Could you check a few things on this drawing? It's one solid part, dimensions in mm from its lowest x, y, z. Round coordinates to 2 decimals unless told otherwise and drop trailing zeros. Loops run counter-clockwise (first coordinate to the right, second up) from the corner with the lowest first, then second, coordinate; pieces in that order, holes last. Notation, with made-up numbers: (-32, 88.25) -> (-16, 88.25) arc R33 cw to (-16, 122.25) -> close; hole circle Ø10 at (30, 29.25). An arc over 180 degrees is marked (long way). Use one line per item in the form item = value. Start each with the question number.
Item 1: If I drill on L1, parallel to Y at x = 168, z = 8; L2, parallel to Y at x = 127.5, z = 19.25, over which ranges is the centre line in solid material (lowest first)? Write a range as [from, to].
Item 2: If we section it at C-C (x = 223): Write out the boundary of the cut face in (y, z), then the cut area to 3 significant figures.
Item 3: If we section it at A-A (y = 20.25): Write out the boundary of the cut face in (x, z).
Item 4: I'm going to push flat-ended pins straight in: pin 1 Ø0.6 at (x, z) = (140, 23.5) entering from +Y; pin 2 Ø6 at (y, z) = (19.5, 14.5) entering from +X. Where does each tip first touch, or does it pass through?
Item 5: If we section it at D-D (y = 4.75): Write out the boundary of the cut face in (x, z).
Item 6: If we section it at B-B (z = 11): Write out the boundary of the cut face in (x, y), then the cut area to 3 significant figures.
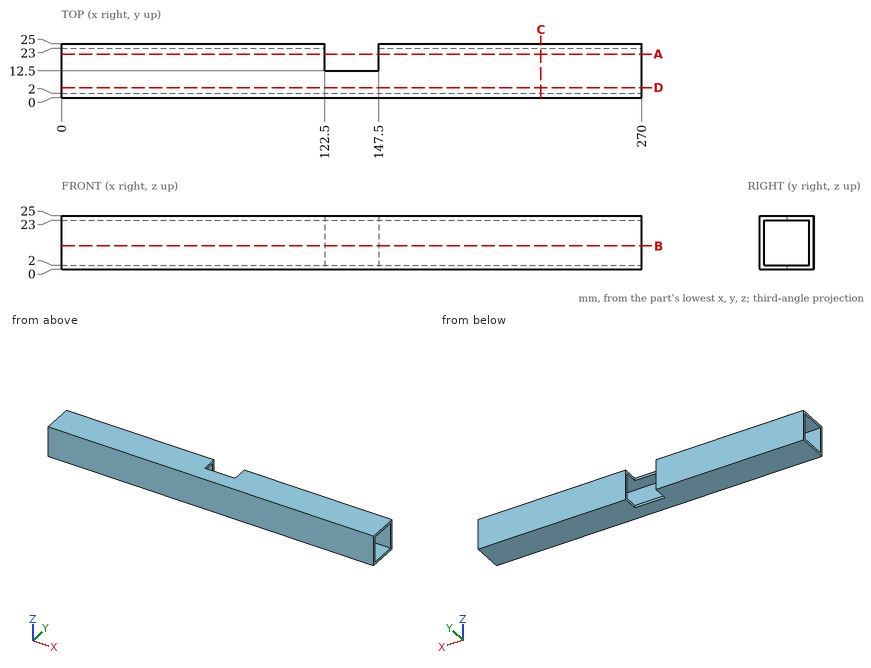
Values found:
q1.L1 = [0, 2], [23, 25]
q1.L2 = [0, 2]
q2.outline = (0, 0) -> (25, 0) -> (25, 25) -> (0, 25) -> close; hole (2, 2) -> (23, 2) -> (23, 23) -> (2, 23) -> close
q2.area = 184 mm2
q3.outline = (0, 0) -> (122.5, 0) -> (122.5, 2) -> (0, 2) -> close; (0, 23) -> (122.5, 23) -> (122.5, 25) -> (0, 25) -> close; (147.5, 0) -> (270, 0) -> (270, 2) -> (147.5, 2) -> close; (147.5, 23) -> (270, 23) -> (270, 25) -> (147.5, 25) -> close
q4.pin_1 = 12.5
q4.pin_2 = through
q5.outline = (0, 0) -> (270, 0) -> (270, 2) -> (0, 2) -> close; (0, 23) -> (270, 23) -> (270, 25) -> (0, 25) -> close
q6.outline = (0, 0) -> (270, 0) -> (270, 2) -> (0, 2) -> close; (0, 23) -> (122.5, 23) -> (122.5, 25) -> (0, 25) -> close; (147.5, 23) -> (270, 23) -> (270, 25) -> (147.5, 25) -> close
q6.area = 1,030 mm2
